Source: three-view drawing plus pictorial views. Frame: mm from the lowest corner of the part. A direction names the side the tool comes from. Give positions to 0.01 mm unless a question says otherwise; leave off trailing zeros. Loops run counter-clockwise (first coordinate to the right, second up) from the corner with the lowest first, then second, coordinate; pieces in that order, holes last. Notation, with made-up numbers: (3, 13) - (10, 13) arc R23 cw to (10, 51) - close; hole circle Ø9 at (-12, 22.5). An arc over 180 degrees is marked (long way). Answer as a JSON object with one key per item and string values.
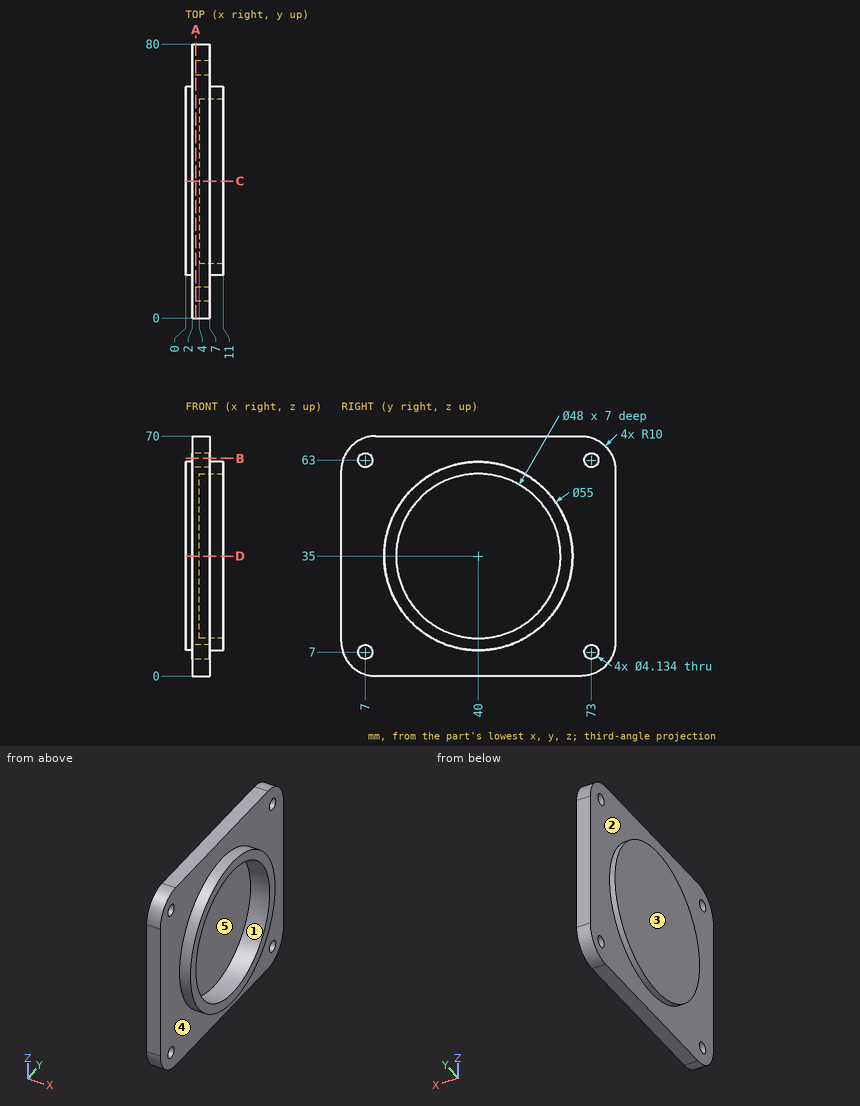
Item 1: Cut plane D-D (z = 35). Return loops of the section in (x, y).
Geometry check:
{"outline": "(0, 12.5) - (2, 12.5) - (2, 0) - (7, 0) - (7, 12.5) - (11, 12.5) - (11, 16) - (4, 16) - (4, 64) - (11, 64) - (11, 67.5) - (7, 67.5) - (7, 80) - (2, 80) - (2, 67.5) - (0, 67.5) - close"}
Item 2: Cut plane A-A (x = 3). Return loops of the section in (y, z).
Geometry check:
{"outline": "(0, 10) arc R10 ccw to (10, 0) - (70, 0) arc R10 ccw to (80, 10) - (80, 60) arc R10 ccw to (70, 70) - (10, 70) arc R10 ccw to (0, 60) - close; hole circle Ø4.13 at (7, 7); hole circle Ø4.13 at (7, 63); hole circle Ø4.13 at (73, 7); hole circle Ø4.13 at (73, 63)"}
Item 3: Material intervals for line 1 (Y direction, x = 3.3, z = 7); line 2 (Y direction, x = 2.5, z = 61.5); line 3 (Z direction, x = 5.2, y = 7), sorted ascending. Write a range as [from, to].
Geometry check:
{"line 1": "y = [0.46, 4.93], [9.07, 70.93], [75.07, 79.54]", "line 2": "y = [0.11, 5.58], [8.42, 71.58], [74.42, 79.89]", "line 3": "z = [0.46, 4.93], [9.07, 60.93], [65.07, 69.54]"}
Item 4: Mould query, pull axis Y, two halves, no side actions, for the marked faces 4 and 5. Classes: released by +Y, released by -Y, zero draft, split by the parting line, or undercut.
Geometry check:
{"face 4": "zero draft", "face 5": "undercut"}
Item 5: Access query for the marked faces 1, 2 and 3. Directions: +Z, -Z, +X, -X, +Y, -Y. A direction counts if a zero-diameter tool reaches every point of the face in a straight line with its end or side. Return the directions, or none.
Geometry check:
{"face 1": "+X", "face 2": "-X", "face 3": "+Z, -Z, -X, +Y, -Y"}
Item 6: Cut plane B-B (z = 63.5). Return loops of the section in (x, y), then the cut area to 3 significant figures.
Geometry check:
{"outline": "(2, 0.63) - (7, 0.63) - (7, 4.99) - (2, 4.99) - close; (2, 9.01) - (7, 9.01) - (7, 70.99) - (2, 70.99) - close; (2, 75.01) - (7, 75.01) - (7, 79.37) - (2, 79.37) - close", "area": "354 mm2"}
Item 7: Cut plane C-C (y = 40). Return loops of the section in (x, z).
Geometry check:
{"outline": "(0, 7.5) - (2, 7.5) - (2, 0) - (7, 0) - (7, 7.5) - (11, 7.5) - (11, 11) - (4, 11) - (4, 59) - (11, 59) - (11, 62.5) - (7, 62.5) - (7, 70) - (2, 70) - (2, 62.5) - (0, 62.5) - close"}
Item 8: Contact query for flat-ended pins moving along their axis: P1, Ø6.5, axis at y = 73, z = 63, coming from the -X side; P2, Ø5, axis at y = 73, z = 7, coming from the +X side; P3, Ø4, axis at y = 46, z = 47, coming from the +X side. Output: stop coordinate, or through.
Geometry check:
{"P1": "stops at x = 2", "P2": "stops at x = 7", "P3": "stops at x = 4"}
